For this review, take the finished solid that the model builds, in its own axes (mm). A direction names the side the tool comes from. Coordinates: 2 decimals unless noted, no trailing zeros. Order: outer loops, then holes, each group sorted by start corner. A loop starts at its lowest first (then second) coordinate and runs counter-clockwise, first axis right, second up. Notation, with made-up numbers: (68.25, 3) - (127.25, 3) arc R28 cw to (127.25, 41) - close; hole circle Ø7 at (65, 51). An arc over 180 degrees is marked (long way). One line per item, written item: value. Start each with the question number.
(1) Consider section B-B on y = -91. Write out the cut boundary in (x, z), then the cut area to 3 significant figures.
(2) For faces 1 (the cylindrical face through (51.145, 5.835, 4.948)), 2 (the flat face through (97.52, -25.45, -0.99)), 3 (the flat face through (105, -27, -2)), 4 (the flat face through (100, -145.44, 3)), 5 (the flat face through (93, -28, -1)), list the 3-axis set-ups (+Z, -Z, +X, -X, +Y, -Y) from which the entire face can be reached by the end or side of a thin tool; tool diameter is ignored.
(3) Mouldability with a two-part tool opening along X and no side actions: class faces 6 (the cylindrical face through (85.19, 3.94, 4.95)), 7 (the flat face through (28, -69.24, 3)), 8 (the flat face through (10, -26, 3)) as released by +X, released by -X, zero draft, split by the parting line, or undercut.
(4) Consider section C-C on x = 87.5. Write out the cut boundary in (y, z).
(5) To check wall thickness, follow line 1 along Y through (x, z) = (159, 2.5); line 2 along Y through (x, z) = (67.5, 0.5); line 3 along X through (y, z) = (-106, 0.75). State the ranges of each line that lie inside material, in increasing order.
(6) Clearance check with flat-ended pins moving along their axes: pin 1 (5 mm diameter, centred on x = 116.75, y = 5, fed in from -Z); pin 2 (6.5 mm diameter, centred on x = 185, y = -58.74, fed in from +Z); pin 3 (3 mm diameter, centred on x = 57.35, y = -96.84, fed in from -Z); pin 4 (2.5 mm diameter, centred on y = -117, z = 1, fed in from +X). State where each tip first meets the part, or that it passes through.
(7) Consider section A-A on x = 33.5. Write out the cut boundary in (y, z).
```python
from build123d import *

# Parameters (mm, degrees)
BOSS_EXTRUDE1_DEPTH                            = 6.35
CBORE_FOR_4_SOCKET_HEAD_CAP_SCREW1_D           = 3.2639
CBORE_FOR_4_SOCKET_HEAD_CAP_SCREW1_CBORE_D     = 5.55752
CBORE_FOR_4_SOCKET_HEAD_CAP_SCREW1_CBORE_DEPTH = 2.8448
BOSS_EXTRUDE2_DEPTH                            = 2
BOSS_EXTRUDE3_DEPTH                            = 6.35
CUT_EXTRUDE1_DEPTH                             = 3


with BuildPart() as part:
    # Outline → Boss-Extrude1 (new body)
    with BuildSketch(Plane.XY):
        Polygon((10, -63.74011537), (52.353553391, -63.74011537), (52.353553391, -139.94011537), (148.353553391, -139.94011537), (148.353553391, -63.74011537), (190, -63.74011537), (190, 10), (10, 10), align=None)
    extrude(amount=BOSS_EXTRUDE1_DEPTH)

    # CBORE for #4 Socket Head Cap Screw1 (through all)
    with Locations(Plane(origin=(14.3688, 5, 6.35), x_dir=(1, 0, 0), z_dir=(0, 0, 1))):
        with Locations((0, 0), (0, -63.74011537), (42.984753391, -63.74011537), (34.12624, 0), (68.25248, 0), (102.37872, 0), (136.50496, 0), (128.984753391, -63.74011537), (128.984753391, -101.84011537), (42.984753391, -139.94011537), (42.984753391, -101.84011537), (170.6312, -63.74011537), (170.6312, 0), (85.984753391, -139.94011537), (128.984753391, -139.94011537)):
            CounterBoreHole(CBORE_FOR_4_SOCKET_HEAD_CAP_SCREW1_D / 2, CBORE_FOR_4_SOCKET_HEAD_CAP_SCREW1_CBORE_D / 2, CBORE_FOR_4_SOCKET_HEAD_CAP_SCREW1_CBORE_DEPTH)

    # Outline<10> → Boss-Extrude2 (add)
    with BuildSketch(Plane.XY):
        Polygon((128.637824638, -53.74011537), (78.433243174, -3.535533906), (81.96877708, 0), (132.173358544, -50.204581464), align=None)
        Polygon((118.738329701, -53.74011537), (122.273863607, -50.204581464), (72.069282143, 0), (68.533748237, -3.535533906), align=None)
    extrude(amount=-BOSS_EXTRUDE2_DEPTH)

    # Sketch8 → Boss-Extrude3 (add)
    with BuildSketch(Plane.XY):
        Polygon((10, 10), (190, 10), (190, -63.74011537), (148.353553391, -63.74011537), (148.353553391, -139.94011537), (52.353553391, -139.94011537), (52.353553391, -63.74011537), (10, -63.74011537), (10, -69.24011537), (46.853553391, -69.24011537), (46.853553391, -145.44011537), (153.853553391, -145.44011537), (153.853553391, -69.24011537), (195.5, -69.24011537), (195.5, 15.5), (10, 15.5), align=None)
    extrude(amount=BOSS_EXTRUDE3_DEPTH)

    # Sketch8<5> → Cut-Extrude1 (cut)
    with BuildSketch(Plane.XY):
        Polygon((190, 10), (0, 10), (0, 13.5), (193.5, 13.5), (193.5, -67.24011537), (151.853553391, -67.24011537), (151.853553391, -143.44011537), (48.853553391, -143.44011537), (48.853553391, -67.24011537), (0, -67.24011537), (0, -63.74011537), (52.353553391, -63.74011537), (52.353553391, -139.94011537), (148.353553391, -139.94011537), (148.353553391, -63.74011537), (190, -63.74011537), align=None)
        Polygon((52.853553391, -63.24011537), (0, -63.24011537), (0, -63.74011537), (52.353553391, -63.74011537), (52.353553391, -139.94011537), (148.353553391, -139.94011537), (148.353553391, -63.74011537), (190, -63.74011537), (190, 10), (0, 10), (0, 9.5), (189.5, 9.5), (189.5, -63.24011537), (147.853553391, -63.24011537), (147.853553391, -139.44011537), (52.853553391, -139.44011537), align=None)
    extrude(amount=CUT_EXTRUDE1_DEPTH, mode=Mode.SUBTRACT)


solid = part.part
```
Geometry check:
1. outline: (46.85, 0) - (48.85, 0) - (48.85, 3) - (52.85, 3) - (52.85, 0) - (147.85, 0) - (147.85, 3) - (151.85, 3) - (151.85, 0) - (153.85, 0) - (153.85, 6.35) - (46.85, 6.35) - close
1. area: 655 mm^2
2. face 1: +Z
2. face 2: -Z
2. face 3: -Z, +X, -X, +Y, -Y
2. face 4: +Z, -Z, +X, -X, -Y
2. face 5: -Z, -X, -Y
3. face 6: undercut
3. face 7: zero draft
3. face 8: released by -X
4. outline: (-145.44, 0) - (-143.44, 0) - (-143.44, 3) - (-139.44, 3) - (-139.44, 0) - (-22.5, 0) - (-22.5, -2) - (-15.43, -2) - (-15.43, 0) - (-12.6, 0) - (-12.6, -2) - (-5.53, -2) - (-5.53, 0) - (9.5, 0) - (9.5, 3) - (13.5, 3) - (13.5, 0) - (15.5, 0) - (15.5, 6.35) - (-145.44, 6.35) - close
5. line 1: y = -69.24 to -67.24, -63.24 to 9.5, 13.5 to 15.5
5. line 2: y = -145.44 to -143.44, -139.44 to 9.5, 13.5 to 15.5
5. line 3: x = 46.85 to 48.85, 52.85 to 147.85, 151.85 to 153.85
6. pin 1: stops at z = 0
6. pin 2: stops at z = 6.35
6. pin 3: passes through
6. pin 4: stops at x = 153.85
7. outline: (-69.24, 0) - (-67.24, 0) - (-67.24, 3) - (-63.24, 3) - (-63.24, 0) - (9.5, 0) - (9.5, 3) - (13.5, 3) - (13.5, 0) - (15.5, 0) - (15.5, 6.35) - (-69.24, 6.35) - close
